Job drawing, mm, ordinate dimensions from the low corner. One solid piece. A direction names the side the tool comes from. Round coordinates to 2 decimals unless told otherwise and drop trailing zeros. Loops run counter-clockwise (first coordinate to the right, second up) from the corner with the lowest first, then second, coordinate; pieces in that order, holes last. Notation, with made-up numbers: M 85,36 L 96,36 A16 ccw 96,62 Z; hole C 15,27.5 d5. An arc over 180 degrees is marked long. Use a Markdown table: item, result. Add a question column.
(1) Band-saw the part on D-D, the plane y = 27. Write the cut outline in (x, z), and give its area (3 significant figures).
(2) Two-plate mould, pull along Y, no slides. Class the marked faces 1, 2 and 3: released by +Y, released by -Y, zero draft, split by the parting line, or undercut.
(3) Band-saw the part on A-A, the plane x = 11.75. Write the cut outline in (y, z).
(4) Which spindle directions (+Z, -Z, +X, -X, +Y, -Y) get a long thin tool onto all of the face, cutting with end or side? Do the marked faces 4, 5 and 6. Say none if no direction does.
(5) Wall check: L1, parallel to X at y = 70, z = 3.8; L2, parallel to Z at x = 18.2, y = 15; L3, parallel to Z at x = 14, y = 4.5. Give the ranges that are in metal, low to high.
(6) Flat gauge pins, fed straight in: P1, Ø2.5, axis at x = 18.5, z = 12.5, coming from the +Y side; P2, Ø5, axis at x = 6.5, z = 6.5, coming from the +Y side; P3, Ø2, axis at x = 17.5, z = 26, coming from the -Y side. Where does each tip first touch, or does it go through?
(7) Band-saw the part on B-B, the plane y = 69. Write the cut outline in (x, z).
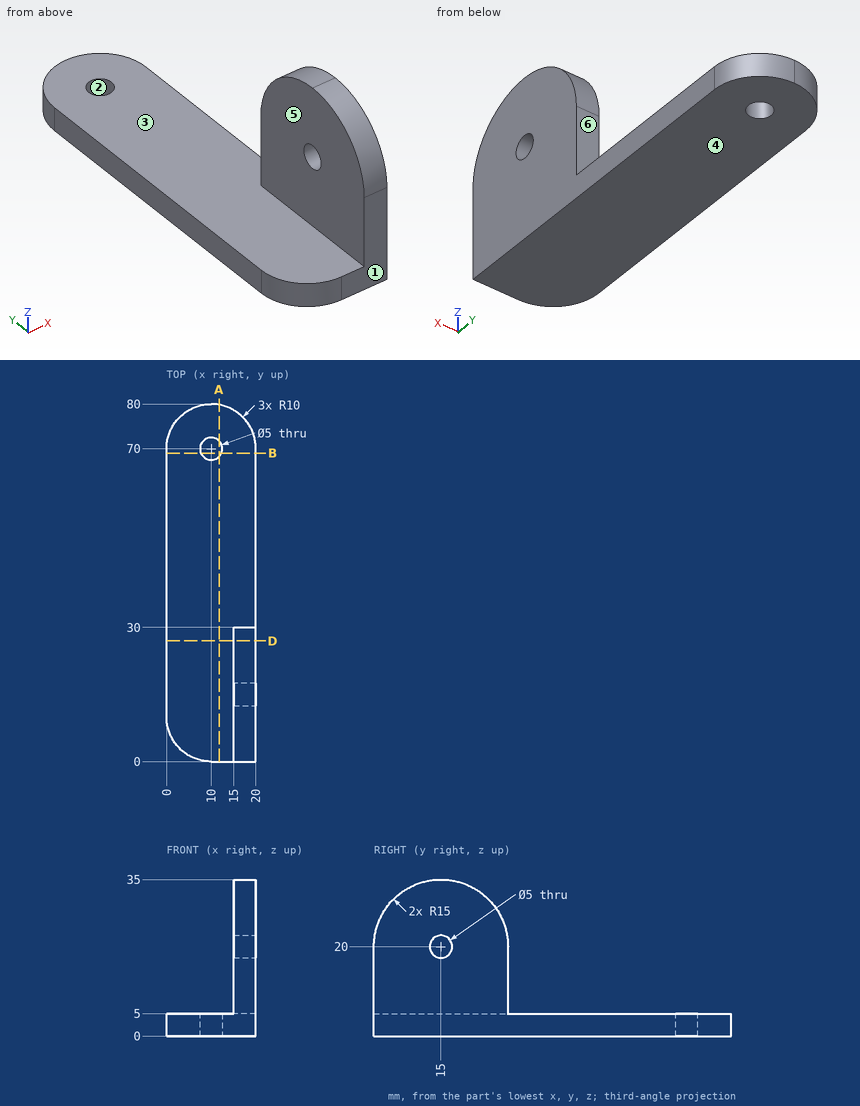
Return value:
| question | item | result |
|---|---|---|
| 1 | outline | M 0,0 L 20,0 L 20,29 L 15,29 L 15,5 L 0,5 Z |
| 1 | area | 220 mm^2 |
| 2 | face 1 | released by -Y |
| 2 | face 2 | undercut |
| 2 | face 3 | zero draft |
| 3 | outline | M 0,0 L 68.21,0 L 68.21,5 L 0,5 Z; M 71.79,0 L 79.85,0 L 79.85,5 L 71.79,5 Z |
| 4 | face 4 | -Z, +X, -X, +Y, -Y |
| 4 | face 5 | +Z, -X, +Y, -Y |
| 4 | face 6 | +Z, +X, -X, +Y |
| 5 | L1 | 0 to 7.5, 12.5 to 20 |
| 5 | L2 | 0 to 17.5, 22.5 to 35 |
| 5 | L3 | 0 to 5 |
| 6 | P1 | y = 30 |
| 6 | P2 | y = 79.89 |
| 6 | P3 | y = 0.86 |
| 7 | outline | M 0,0 L 7.71,0 L 7.71,5 L 0,5 Z; M 12.29,0 L 20,0 L 20,5 L 12.29,5 Z |
